from build123d import *

# Parameters (mm, degrees)
SKIZZE1_W                       = 18
SKIZZE1_H                       = 1.3
SKIZZE1_H_2                     = 1.4
SKIZZE1_H_3                     = 2
SKIZZE1_H_4                     = 28.3
SKIZZE1_R                       = 1.55
AUFSATZ_LINEAR_AUSTRAGEN3_DEPTH = 5
SKIZZE1_4_W                     = 18
SKIZZE1_4_H                     = 1.3
SKIZZE1_4_H_2                   = 2
AUFSATZ_LINEAR_AUSTRAGEN4_DEPTH = 6
SKIZZE2_W                       = 2
SKIZZE2_H                       = 9
SCHNITT_LINEAR_AUSTRAGEN1_DEPTH = 29.674901918


with BuildPart() as part:
    # Skizze1 → Aufsatz-Linear austragen3 (new body)
    # profile 1 of 4: a face of its own
    with BuildSketch(Plane.XY):
        with Locations((0, 20.85)):
            Rectangle(SKIZZE1_W, SKIZZE1_H)
    # profile 2 of 4: a face of its own
    with BuildSketch(Plane.XY):
        with Locations((0, 19.5)):
            Rectangle(SKIZZE1_W, SKIZZE1_H_2)
    # profile 3 of 4: a face of its own
    with BuildSketch(Plane.XY):
        with Locations((0, 17.8)):
            Rectangle(SKIZZE1_W, SKIZZE1_H_3)
    # profile 4 of 4: a face of its own
    with BuildSketch(Plane.XY):
        with Locations((0, 2.65)):
            Rectangle(SKIZZE1_W, SKIZZE1_H_4)
        with Locations((-5, -7.5)):
            Circle(SKIZZE1_R, mode=Mode.SUBTRACT)
        with Locations((5, -7.5)):
            Circle(SKIZZE1_R, mode=Mode.SUBTRACT)
        with Locations((-5, 7.5)):
            Circle(SKIZZE1_R, mode=Mode.SUBTRACT)
        with Locations((5, 7.5)):
            Circle(SKIZZE1_R, mode=Mode.SUBTRACT)
    extrude(amount=-AUFSATZ_LINEAR_AUSTRAGEN3_DEPTH)

    # Skizze1_4 → Aufsatz-Linear austragen4 (add)
    with BuildSketch(Plane.XY):
        with Locations((0, 20.85)):
            Rectangle(SKIZZE1_4_W, SKIZZE1_4_H)
        with Locations((0, 17.8)):
            Rectangle(SKIZZE1_4_W, SKIZZE1_4_H_2)
    extrude(amount=AUFSATZ_LINEAR_AUSTRAGEN4_DEPTH)

    # Skizze2 → Schnitt-Linear austragen1 (cut, through all)
    with BuildSketch(Plane(origin=(9, 0, 0), x_dir=(0, 0, -1), z_dir=(1, 0, 0))):
        with Locations((4, 17)):
            Rectangle(SKIZZE2_W, SKIZZE2_H)
    extrude(amount=-SCHNITT_LINEAR_AUSTRAGEN1_DEPTH, mode=Mode.SUBTRACT)


solid = part.part
Geometry check sheet. Reference: the model listing, model coordinates, mm. A direction names the side the tool comes from. Coordinates: 2 decimals unless noted, no trailing zeros. Order: outer loops, then holes, each group sorted by start corner. A loop starts at its lowest first (then second) coordinate and runs counter-clockwise, first axis right, second up. Notation, with made-up numbers: M 0,-19 L 43,-19 A17 cw 43,2 Z; hole C -13,73 d7. An arc over 180 degrees is marked long. Use CSV: the item, a comma, the result in double quotes.
Item 1: Gauge pin test, flat ends, axial feed: pin 1 Ø4.5 at (x, y) = (-3.5, 17) entering from -Z; pin 2 Ø1.5 at (x, y) = (4.5, -3.5) entering from +Z; pin 3 Ø1.8 at (x, z) = (0.5, 4.5) entering from -Y. Record the tip position at first contact, or that the pin passes through.
Returned:
pin 1,"stops at z = -3"
pin 2,"stops at z = 0"
pin 3,"stops at y = 16.8"
Item 2: Tool access check on faces 1 (the flat face through (0, 16.8, 3)), 2 (the flat face through (0, 18.8, 3)), 3 (the flat face through (0, -11.5, -2)), 4 (the flat face through (0, 12.5, -4)). Record the directions out of +Z, -Z, +X, -X, +Y, -Y that give a thin tool (end or side, any length) a straight path to the whole face; none if there is none.
Returned:
face 1,"+Z, +X, -X, -Y"
face 2,"+Z, +X, -X"
face 3,"+Z, -Z, +X, -X, -Y"
face 4,"-Z, +X, -X, +Y"
Item 3: Cross-section at D-D on z = 2. Record the cut outline in (x, y).
Returned:
outline,"M -9,16.8 L 9,16.8 L 9,18.8 L -9,18.8 Z; M -9,20.2 L 9,20.2 L 9,21.5 L -9,21.5 Z"
Item 4: Cross-section at A-A on y = -7.5. Record the cut outline in (x, z).
Returned:
outline,"M -9,-5 L -6.55,-5 L -6.55,0 L -9,0 Z; M -3.45,-5 L 3.45,-5 L 3.45,0 L -3.45,0 Z; M 6.55,-5 L 9,-5 L 9,0 L 6.55,0 Z"
Item 5: Cross-section at B-B on x = -5. Record the cut outline in (y, z), then the cut area to 3 significant figures.
Returned:
outline,"M -11.5,-5 L -9.05,-5 L -9.05,0 L -11.5,0 Z; M -5.95,-5 L 5.95,-5 L 5.95,0 L -5.95,0 Z; M 9.05,-5 L 12.5,-5 L 12.5,-3 L 21.5,-3 L 21.5,6 L 20.2,6 L 20.2,0 L 18.8,0 L 18.8,6 L 16.8,6 L 16.8,0 L 9.05,0 Z"
area,"136 mm2"
Item 6: Cross-section at C-C on z = -1. Record the cut outline in (x, y), then the cut area to 3 significant figures.
Returned:
outline,"M -9,-11.5 L 9,-11.5 L 9,21.5 L -9,21.5 Z; hole C -5,-7.5 d3.1; hole C -5,7.5 d3.1; hole C 5,-7.5 d3.1; hole C 5,7.5 d3.1"
area,"564 mm2"
Item 7: Thickness scan on line 1 along Y through (x, z) = (-5, -3.5); line 2 along Y through (x, z) = (5, -1); line 3 along Y through (x, z) = (-2.5, 3.5). Record the ranges inside material, lowest first.
Returned:
line 1,"y = -11.5 to -9.05, -5.95 to 5.95, 9.05 to 12.5"
line 2,"y = -11.5 to -9.05, -5.95 to 5.95, 9.05 to 21.5"
line 3,"y = 16.8 to 18.8, 20.2 to 21.5"
